from build123d import *

# Parameters (mm, degrees)
SKETCH_R      = 27.5
SKETCH_R_2    = 17.5
PAD_DEPTH     = 25
SKETCH001_R   = 17.5
SKETCH001_R_2 = 4.55
SKETCH001_R_3 = 1.5
PAD001_DEPTH  = 16
SKETCH002_R   = 17.5
POCKET_DEPTH  = 13
SKETCH003_R   = 5.55
SKETCH003_R_2 = 4.55
PAD002_DEPTH  = 2
SKETCH004_R   = 5.55
SKETCH004_R_2 = 4.55
PAD003_DEPTH  = 2


with BuildPart() as part:
    # Sketch → Pad (new body)
    with BuildSketch(Plane.YZ):
        Circle(SKETCH_R)
        Circle(SKETCH_R_2, mode=Mode.SUBTRACT)
    extrude(amount=-PAD_DEPTH)

    # Sketch001 → Pad001 (join)
    with BuildSketch(Plane.YZ):
        Circle(SKETCH001_R)
        Circle(SKETCH001_R_2, mode=Mode.SUBTRACT)
        with Locations((0, 10)):
            Circle(SKETCH001_R_3, mode=Mode.SUBTRACT)
        with Locations((-8.660254, -5)):
            Circle(SKETCH001_R_3, mode=Mode.SUBTRACT)
        with Locations((8.660254, -5)):
            Circle(SKETCH001_R_3, mode=Mode.SUBTRACT)
    extrude(amount=-PAD001_DEPTH)

    # Sketch002 → Pocket (cut)
    with BuildSketch(Plane.YZ):
        Circle(SKETCH002_R)
    extrude(amount=-POCKET_DEPTH, mode=Mode.SUBTRACT)

    # Sketch003 (on Face6 of Pocket) → Pad002 (join)
    with BuildSketch(Plane.YZ.offset(-13)):
        Circle(SKETCH003_R)
        Circle(SKETCH003_R_2, mode=Mode.SUBTRACT)
    extrude(amount=PAD002_DEPTH)

    # Sketch004 (on Face7 of Pad002) → Pad003 (join)
    with BuildSketch(Plane(origin=(-16, 0, 0), x_dir=(0, 1, 0), z_dir=(-1, 0, 0))):
        Circle(SKETCH004_R)
        Circle(SKETCH004_R_2, mode=Mode.SUBTRACT)
    extrude(amount=PAD003_DEPTH)


solid = part.part
Geometry: final body of the model. Coordinates: model frame, mm. A direction names the side the tool comes from. Round coordinates to 2 decimals unless told otherwise and drop trailing zeros. Write each loop counter-clockwise with the first axis right and the second up, starting at its lowest first coordinate (ties: lowest second). Pieces come first, ordered by that corner, then holes. Notation, with made-up numbers: M -9,10.25 L 49,10.25 A25 ccw 49,32.25 Z; hole C 56,7 d11. An arc over 180 degrees is marked long. Write item = value, one per line.
Item 1: Section query C-C on x = -14.75. Return loops of the section in (y, z).
Findings:
outline = C 0,0 d55; hole C -8.66,-5 d3; hole C 0,0 d9.1; hole C 0,10 d3; hole C 8.66,-5 d3
Item 2: Pin query (flat end, axial travel): P1, Ø8, axis at x = -20, y = 10, coming from the -Z side; P2, Ø3, axis at y = 8, z = -5, coming from the +X side; P3, Ø4, axis at x = -3.5, y = 5, coming from the +Z side; P4, Ø7.5, axis at y = 0, z = 0, coming from the +X side. Return the tip coordinate at first contact, or that it passes through.
Findings:
P1 = -26.84
P2 = -13
P3 = 27.34
P4 = through
Item 3: Pull-direction query (Z, two-part tool) for faces 4 (the face through (-12.01, 2.98, 4.68)), 5 (the face through (0, 0, -18)), 6 (the face through (-12.325, -5.961, -26.846)); classes: pulls with the +Z half, pulls with the -Z half, needs draft (parallel to the pull), parting line crosses it, or undercut.
Findings:
face_4 = undercut
face_5 = needs draft
face_6 = parting line crosses it
Item 4: Section query B-B on z = 10. Return loops of the section in (x, y), then the cut area to 3 significant figures.
Findings:
outline = M -25,-25.62 L 0,-25.62 L 0,-14.36 L -13,-14.36 L -13,-1.5 L -16,-1.5 L -16,-14.36 L -25,-14.36 Z; M -25,14.36 L -16,14.36 L -16,1.5 L -13,1.5 L -13,14.36 L 0,14.36 L 0,25.62 L -25,25.62 Z
area = 640 mm^2
Item 5: Section query A-A on y = 0. Return loops of the section in (x, z).
Findings:
outline = M -25,-27.5 L 0,-27.5 L 0,-17.5 L -13,-17.5 L -13,-5.55 L -11,-5.55 L -11,-4.55 L -18,-4.55 L -18,-5.55 L -16,-5.55 L -16,-17.5 L -25,-17.5 Z; M -25,17.5 L -16,17.5 L -16,11.5 L -13,11.5 L -13,17.5 L 0,17.5 L 0,27.5 L -25,27.5 Z; M -18,4.55 L -11,4.55 L -11,5.55 L -13,5.55 L -13,8.5 L -16,8.5 L -16,5.55 L -18,5.55 Z
Item 6: Material intervals for line 1 along Z through (x, y) = (-15.25, 0); line 2 along Z through (x, y) = (-1, -0.5); line 3 along Y through (x, z) = (-13.25, -4), sorted ascending. Write a range as [from, to].
Findings:
line_1 = [-27.5, -4.55], [4.55, 8.5], [11.5, 27.5]
line_2 = [-27.5, -17.49], [17.49, 27.5]
line_3 = [-27.21, -9.78], [-7.54, -2.17], [2.17, 7.54], [9.78, 27.21]
Item 7: Access query for faces 1 (the face through (-18, 0, -5)), 2 (the face through (-11, 0, 5)), 3 (the face through (-14.45, -0.99, 4.44)). Directions: +Z, -Z, +X, -X, +Y, -Y. A direction counts if a zero-diameter tool reaches every point of the face in a straight line with its end or side. Return the directions, or none.
Findings:
face_1 = -X
face_2 = +X
face_3 = +X, -X
Item 8: Section query D-D on y = 11.5. Return loops of the section in (x, z), then the cut area to 3 significant figures.
Findings:
outline = M -25,-24.98 L 0,-24.98 L 0,-13.19 L -13,-13.19 L -13,13.19 L 0,13.19 L 0,24.98 L -25,24.98 L -25,13.19 L -16,13.19 L -16,-13.19 L -25,-13.19 Z
area = 669 mm^2
